Design review of the part built by this model. Coordinates are the model's own, in mm. A direction names the side the tool comes from. Coordinates: 2 decimals unless noted, no trailing zeros. Write each loop counter-clockwise with the first axis right and the second up, starting at its lowest first coordinate (ties: lowest second). Pieces come first, ordered by that corner, then holes.
Q1. Take a section at A-A (x = 11.25). Give the boundary of the cut face in (y, z), and give its area (3 significant figures).
Q2. Take a section at B-B (y = 12.5). Give the boundary of the cut face in (x, z).
Q3. Machinability: for faces 1 (the flat face through (1, 13, 152.4)), 2 (the flat face through (13, 23.818, 75)), which of the approach directions +Z, -Z, +X, -X, +Y, -Y give a long, thin tool a straight path to every point of the face, cutting with its end or side? Answer none if there is none.
Q4. Mouldability with a two-part tool opening along X and no side actions: class faces 3 (the flat face through (13, 0, 75)), 4 (the flat face through (25.4, 13, 75)), 5 (the flat face through (1.588, 13, 75)) as pulls with the +X half, pulls with the -X half, needs draft (parallel to the pull), parting line crosses it, or undercut.
Q5. For probe 1 along Y at (x, z) = (18.5, 60); probe 2 along X at (y, z) = (22.25, 103.5), list the stretches that pass through material, from the lowest coordinate up.
Q6. Take a section at C-C (z = 77). Give the boundary of the cut face in (x, y).
Autodesk Inventor part; units mm, degrees
ref_plane "YZ Plane" through (0, 0, 0) normal (1, 0, 0) x (0, 1, 0)
ref_plane "XZ Plane" through (0, 0, 0) normal (0, 1, 0) x (-1, 0, 0)
ref_plane "XY Plane" through (0, 0, 0) normal (0, 0, 1) x (1, 0, 0)
sketch "Sketch1" plane through (0, 0, 0) normal (0, 0, 1) x (1, 0, 0)
  line L0 (0, 0) -> (25.4, 0)
  line L1 (25.4, 0) -> (25.4, 25.4053)
  line L2 (25.4, 25.4053) -> (0, 25.4053)
  line L3 (0, 25.4053) -> (0, 0)
  line L4 (1.5875, 22.2862) -> (1.5875, 23.8178) construction
  line L5 (1.5875, 23.8178) -> (23.8125, 23.8178)
  line L6 (23.8125, 23.8178) -> (23.8125, 1.5875)
  line L7 (23.8125, 1.5875) -> (1.5875, 1.5875)
  line L8 (1.5875, 1.5875) -> (1.5875, 23.8178)
  dimension "d0" = 25.4
  dimension "d4" = 22.225
extrude "Extrusion1" add sketch "Sketch1" along normal blind 152.4
properties part number "Hook 2nd 1x1"
Response:
1. outline: (0, 0) - (1.59, 0) - (1.59, 152.4) - (0, 152.4) - close; (23.82, 0) - (25.41, 0) - (25.41, 152.4) - (23.82, 152.4) - close
1. area: 484 mm2
2. outline: (0, 0) - (1.59, 0) - (1.59, 152.4) - (0, 152.4) - close; (23.81, 0) - (25.4, 0) - (25.4, 152.4) - (23.81, 152.4) - close
3. face 1: +Z, +X, -X, +Y, -Y
3. face 2: +Z, -Z
4. face 3: needs draft
4. face 4: pulls with the +X half
4. face 5: undercut
5. probe 1: y = 0 to 1.59, 23.82 to 25.41
5. probe 2: x = 0 to 1.59, 23.81 to 25.4
6. outline: (0, 0) - (25.4, 0) - (25.4, 25.41) - (0, 25.41) - close; hole (1.59, 1.59) - (23.81, 1.59) - (23.81, 23.82) - (1.59, 23.82) - close
